Check sheet for the drawn part. Datum: minimum x, y, z corner. Units: mm. A direction names the side the tool comes from. Round coordinates to 2 decimals unless told otherwise and drop trailing zeros. Write each loop counter-clockwise with the first axis right and the second up, starting at its lowest first coordinate (ties: lowest second). Pieces come first, ordered by that corner, then holes. Notation, with made-up numbers: (80, 3.25) - (104, 3.25) arc R23 ccw to (104, 39.25) - close; hole circle Ø1 at (72, 81). An arc over 180 degrees is marked (long way). Write each question's results on one line, items separated by ' | '.
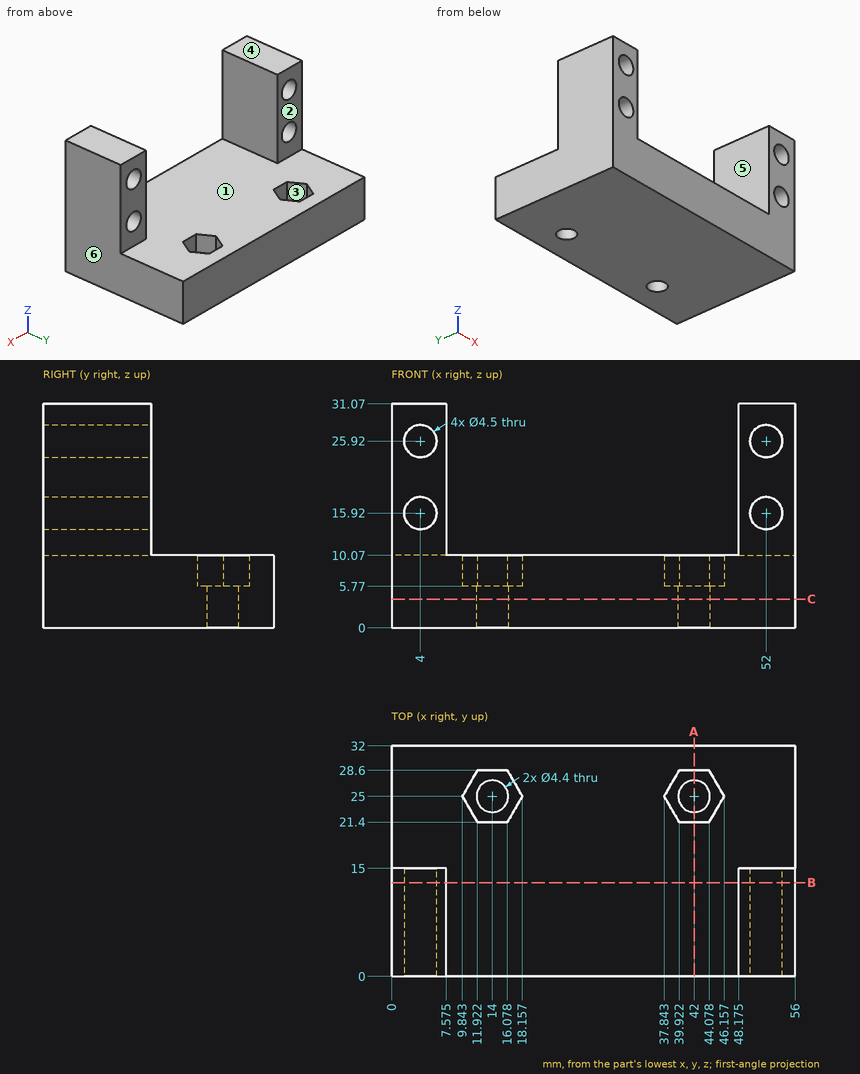
(1) Thickness scan on L1, parallel to Z at x = 52, y = 6; L2, parallel to X at y = 11, z = 21 (1 decimal); L3, parallel to Y at x = 14, z = 2.3. Record the ranges inside material, lowest first.
Answer:
L1: 0 to 13.67, 18.17 to 23.67, 28.17 to 31.07 | L2: 0 to 7.6, 48.2 to 56 | L3: 0 to 22.8, 27.2 to 32
(2) Go/stop test with flat-tipped pins: pin 1 Ø7 at (x, z) = (4, 25.92) entering from +Y; pin 2 Ø2 at (x, y) = (25.5, 10) entering from +Z; pin 3 Ø5.5 at (x, y) = (14, 25) entering from +Z. Record where each tip stops, or that it passes through.
Answer:
pin 1: y = 15 | pin 2: z = 10.07 | pin 3: z = 5.77
(3) Section check A-A (x = 42). Record the cut outline in (y, z), plus the area to 3 significant figures.
Answer:
outline: (0, 0) - (22.8, 0) - (22.8, 5.77) - (21.4, 5.77) - (21.4, 10.07) - (0, 10.07) - close; (27.2, 0) - (32, 0) - (32, 10.07) - (28.6, 10.07) - (28.6, 5.77) - (27.2, 5.77) - close | area: 266 mm2
(4) Mould release check, pull along X, two halves, no side actions. Record for the marked faces 4, 5 and 6: released by +X, released by -X, zero draft, split by the parting line, or undercut.
Answer:
face 4: zero draft | face 5: undercut | face 6: released by +X
(5) Section check B-B (y = 13). State how many separate pieces and enclosed holes the cut face has.
Answer:
separate pieces: 1 | enclosed holes: 4
(6) Set-up check for the marked faces 1, 2 and 3: record each of +Z, -Z, +X, -X, +Y, -Y from which the full face is reachable in a straight line by a thin tool's end or side.
Answer:
face 1: +Z, +Y | face 2: +Z, +X, -X, +Y | face 3: +Z
(7) Section check C-C (z = 4). Record the cut outline in (x, y), plus the area to 3 significant figures.
Answer:
outline: (0, 0) - (56, 0) - (56, 32) - (0, 32) - close; hole circle Ø4.4 at (14, 25); hole circle Ø4.4 at (42, 25) | area: 1,760 mm2
